Geometry check sheet. Reference: the model listing, model coordinates, mm. Face numbers are marked on the shaded views. A direction names the side the tool comes from. Coordinates: 2 decimals unless noted, no trailing zeros. Write each loop counter-clockwise with the first axis right and the second up, starting at its lowest first coordinate (ties: lowest second). Pieces come first, ordered by that corner, then holes. Notation, with made-up numbers: (-19, 5) -> (-5, 5) arc R31 cw to (-5, 42) -> close; hole circle Ø11 at (12.5, 23). An arc over 180 degrees is marked (long way). Put each result on its own line as item: value. Start each with the question number.
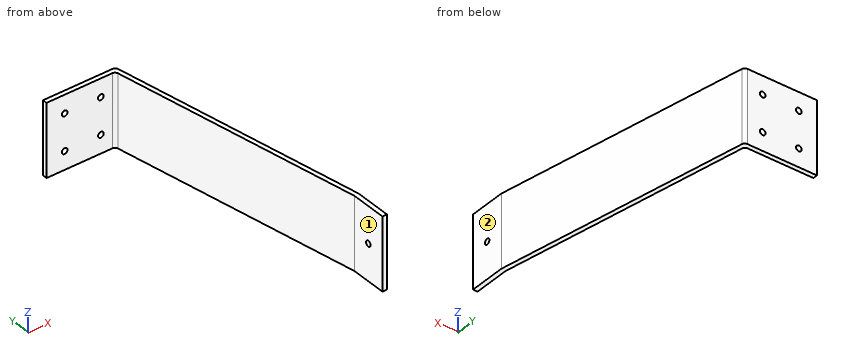
from build123d import *

# Parameters (mm, degrees)
BOSS_EXTRUDE1_DEPTH = 25.4
SKETCH3_R           = 2
CUT_EXTRUDE1_DEPTH  = 50.8
SKETCH4_R           = 2
CUT_EXTRUDE2_DEPTH  = 83.15093717
FILLET1_R           = 2.38


with BuildPart() as part:
    # Sketch1 → Boss-Extrude1 (new body, symmetric)
    with BuildSketch(Plane.XY):
        Polygon((0, 0), (50.8, 0), (82.15093717, -177.8), (82.15093717, -203.2), (78.97593717, -203.2), (78.97593717, -178.077776507), (48.135858671, -3.175), (0, -3.175), align=None)
    extrude(amount=BOSS_EXTRUDE1_DEPTH, both=True)

    # Sketch3 → Cut-Extrude1 (cut)
    with BuildSketch(Plane(origin=(0, 0, 0), x_dir=(1, 0, 0), z_dir=(0, 1, 0))):
        with Locations((12.7, -12.7)):
            Circle(SKETCH3_R)
        with Locations((12.7, 12.7)):
            Circle(SKETCH3_R)
        with Locations((38.1, 12.7)):
            Circle(SKETCH3_R)
        with Locations((38.1, -12.7)):
            Circle(SKETCH3_R)
    extrude(amount=-CUT_EXTRUDE1_DEPTH, mode=Mode.SUBTRACT)

    # Sketch4 → Cut-Extrude2 (cut, through all)
    with BuildSketch(Plane(origin=(82.15093717, 0, 0), x_dir=(0, 0, -1), z_dir=(1, 0, 0))):
        with Locations((0, -190.5)):
            Circle(SKETCH4_R)
    extrude(amount=-CUT_EXTRUDE2_DEPTH, mode=Mode.SUBTRACT)

    # Fillet1
    fillet1_edges = [part.edges().sort_by_distance(p)[0] for p in [
        (50.8, 0, 0),
        (48.135858671, -3.175, 0),
    ]]
    fillet(fillet1_edges, radius=FILLET1_R)


solid = part.part
Item 1: Section check A-A, the plane z = 0. Enter the section's corners in (x, y) (3 decimals).
Item 2: Access from +Z, -Z, +X, -X, +Y, -Y to the whole of each face (thin tool, end or side, straight path). Record for the marked faces 1 and 2.
Item 3: Section check B-B, the plane x = 38.1. Enter the section's corners in (y, z) (3 decimals), and give its area (3 significant figures).
Item 4: Scan lines: line 1 along Z through (x, y) = (38.1, -2.35); line 2 along X through (y, z) = (-1.85, -12.7); line 3 along X through (y, z) = (-2.1, -12.7). Record each from-to range of solid material in increasing order. Write a range as [from, to].
Item 5: Go/stop test with flat-tipped pins: P1, Ø3.5, axis at x = 12.7, z = 12.7, coming from the +Y side; P2, Ø7.5, axis at y = -189, z = -4, coming from the -X side; P3, Ø14, axis at x = 22, z = 4, coming from the -Y side (3 decimals); P4, Ø8, axis at y = -147, z = 8.5, coming from the +X side. Record where each tip stops, or that it passes through.
Item 6: Section check D-D, the plane z = 12.7. Enter the section's corners in (x, y) (3 decimals).
Item 7: Section check C-C, the plane y = -190.5. Enter the section's corners in (x, z).
From the geometry:
1. outline: (0, -3.175) -> (46.139, -3.175) arc R2.38 cw to (48.483, -5.142) -> (78.976, -178.078) -> (78.976, -188.5) -> (82.151, -188.5) -> (82.151, -177.8) -> (51.147, -1.967) arc R2.38 ccw to (48.803, 0) -> (0, 0) -> close; (78.976, -203.2) -> (82.151, -203.2) -> (82.151, -192.5) -> (78.976, -192.5) -> close
2. face 1: +Z, -Z, -X, -Y
2. face 2: +Z, -Z, +X, +Y, -Y
3. outline: (-3.175, -25.4) -> (0, -25.4) -> (0, -14.7) -> (-3.175, -14.7) -> close; (-3.175, -10.7) -> (0, -10.7) -> (0, 10.7) -> (-3.175, 10.7) -> close; (-3.175, 14.7) -> (0, 14.7) -> (0, 25.4) -> (-3.175, 25.4) -> close
3. area: 136 mm²
4. line 1: [-25.4, -14.7], [-10.7, 10.7], [14.7, 25.4]
4. line 2: [0, 10.7], [14.7, 36.1], [40.1, 51.12]
4. line 3: [0, 10.7], [14.7, 36.1], [40.1, 51.17]
5. P1: through
5. P2: x = 78.98
5. P3: y = -3.175
5. P4: x = 77.43
6. outline: (0, -3.175) -> (10.7, -3.175) -> (10.7, 0) -> (0, 0) -> close; (14.7, -3.175) -> (36.1, -3.175) -> (36.1, 0) -> (14.7, 0) -> close; (40.1, -3.175) -> (46.139, -3.175) arc R2.38 cw to (48.483, -5.142) -> (78.976, -178.078) -> (78.976, -203.2) -> (82.151, -203.2) -> (82.151, -177.8) -> (51.147, -1.967) arc R2.38 ccw to (48.803, 0) -> (40.1, 0) -> close
7. outline: (78.98, -25.4) -> (82.15, -25.4) -> (82.15, -2) -> (78.98, -2) -> close; (78.98, 2) -> (82.15, 2) -> (82.15, 25.4) -> (78.98, 25.4) -> close
